For this review, take the finished solid that the model builds, in its own axes (mm). Face numbers are marked on the shaded views. A direction names the side the tool comes from. Coordinates: 2 decimals unless noted, no trailing zeros. Write each loop counter-clockwise with the first axis right and the second up, starting at its lowest first coordinate (ties: lowest second). Pieces come first, ordered by that corner, then holes.
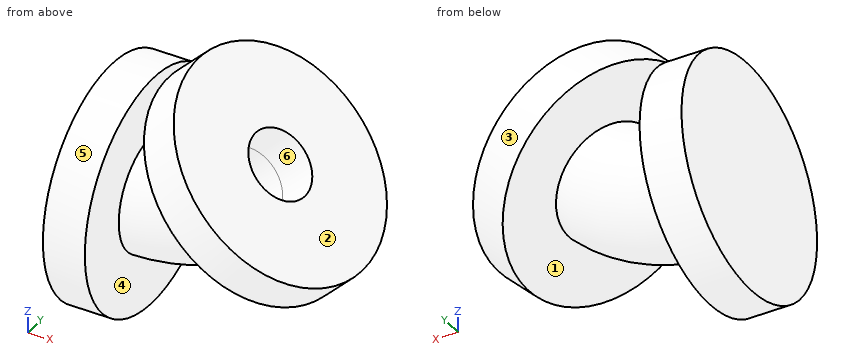
```python
from build123d import *

# Parameters (mm, degrees)
F1_R     = 50
F1_R_2   = 25
F2_DEPTH = 18
F4_R     = 50
F5_DEPTH = 18


with BuildPart() as f2:
    # F1 (on Right) → F2 (new body)
    with BuildSketch(Plane.YZ):
        with Locations((0, -59.5)):
            Circle(F1_R)
        with Locations((0, -59.5)):
            Circle(F1_R_2, mode=Mode.SUBTRACT)
        with Locations((0, -59.5)):
            Circle(F1_R_2)
        with BuildLine():
            ThreePointArc((0, -44.5), (10.6066017178, -48.8933982822), (15, -59.5))
            ThreePointArc((15, -59.5), (-10.6066017178, -70.1066017178), (0, -44.5))
        make_face(mode=Mode.SUBTRACT)
        with BuildLine():
            ThreePointArc((0, -44.5), (-10.6066017178, -70.1066017178), (15, -59.5))
            ThreePointArc((15, -59.5), (10.6066017178, -48.8933982822), (0, -44.5))
        make_face()
    extrude(amount=-F2_DEPTH)

    # F3: sweep along a path in F0
    with BuildLine(Plane.XZ) as f3_path:
        ThreePointArc((0, -59.5), (22.7696642257, -54.9708321844), (42.0728534806, -42.0728534806))
    # F1 (on Right) → F3 (sweep)
    with BuildSketch(Plane.YZ):
        with Locations((0, -59.5)):
            Circle(F1_R_2)
        with BuildLine():
            ThreePointArc((0, -44.5), (10.6066017178, -48.8933982822), (15, -59.5))
            ThreePointArc((15, -59.5), (-10.6066017178, -70.1066017178), (0, -44.5))
        make_face(mode=Mode.SUBTRACT)
    sweep(path=f3_path.line)

    # F4 (on face) → F5 (join)
    with BuildSketch(Plane(origin=(0, 0, 0), x_dir=(0.7071067812, 0, -0.7071067812), z_dir=(0.7071067812, 0, 0.7071067812))):
        with Locations((59.5, 0)):
            Circle(F4_R)
        with BuildLine():
            ThreePointArc((59.5, 15), (70.1066017178, 10.6066017178), (74.5, 0))
            ThreePointArc((74.5, 0), (48.8933982822, -10.6066017178), (59.5, 15))
        make_face(mode=Mode.SUBTRACT)
    extrude(amount=F5_DEPTH)


solid = f2.part
```
1) Clearance check with flat-ended pins moving along their axes: P1, Ø8, axis at y = -30, z = -69.5, coming from the +X side; P2, Ø9, axis at y = -3, z = -57, coming from the +X side; P3, Ø1, axis at x = 36.5, y = -38, coming from the -Z side. State where each tip first meets the part, or that it passes through.
2) Consider section D-D (x = -7). Give the boundary of the cut face in (y, z), then the cut area to 3 significant figures.
3) For L1, parallel to Z at x = 18, y = -7; L2, parallel to X at y = -4.5, z = -97.5; L3, parallel to X at y = -20, z = -31, list the stretches that pass through material, from the lowest coordinate up.
4) The part is to be moulded in two halves that separate along Z. For the marked faces 1, 2, 3 and 4, say which applies: pulls with the +Z half, pulls with the -Z half, needs draft (parallel to the pull), parting line crosses it, or undercut.
5) Consider section B-B (z = -68). Count the separate pieces of the cut face and the enclosed holes in it, then the cut area to 3 significant figures.
6) Consider section A-A (y = -42). Give the boundary of the cut face in (x, z), then the cut area to 3 significant figures.
7) Tool access review of the marked faces 5 and 6: name each direction out of +Z, -Z, +X, -X, +Y, -Y from which nothing blocks a thin tool from reaching the whole face with its end or side.
8) Consider section C-C (y = 2). Give the boundary of the cut face in (x, z), then the cut area to 3 significant figures.
Results:
1. P1: stops at x = 76.84
1. P2: stops at x = 86.96
1. P3: stops at z = -37
2. outline: circle Ø100 at (0, -59.5)
2. area: 7,850 mm2
3. L1: z = -81.54 to -70.51, -42.59 to -30.6, -18 to 3.87
3. L2: x = -18 to 0
3. L3: x = -18 to 0, 31 to 56.46
4. face 1: undercut
4. face 2: pulls with the +Z half
4. face 3: parting line crosses it
4. face 4: needs draft
5. separate pieces: 2
5. enclosed holes: 1
5. area: 3,980 mm2
6. outline: (-18, -86.63) - (0, -86.63) - (0, -32.37) - (-18, -32.37) - close; (22.89, -22.89) - (61.26, -61.26) - (73.98, -48.53) - (35.62, -10.16) - close
6. area: 1,950 mm2
7. face 5: -X
7. face 6: none
8. outline: (-18, -109.46) - (0, -109.46) - (0, -84.42) arc R84.42 ccw to (59.69, -59.69) - (77.4, -77.4) - (90.13, -64.67) - (65.31, -39.86) - (52.58, -52.58) arc R74.37 cw to (0, -74.37) - (0, -44.63) arc R44.63 ccw to (31.56, -31.56) - (44.29, -18.83) - (19.47, 5.98) - (6.75, -6.75) - (24.45, -24.45) arc R34.58 cw to (0, -34.58) - (0, -9.54) - (-18, -9.54) - close
8. area: 4,000 mm2
